from build123d import *

# Parameters (mm, degrees)
SKETCH_R        = 25
PAD_DEPTH       = 25
PAD_TAPER       = 15
SKETCH001_R     = 22.984215
POCKET_DEPTH    = 17
POCKET_TAPER    = 15
SKETCH002_R     = 16.714516
PAD001_DEPTH    = 30
PAD001_TAPER    = 20
SKETCH003_R     = 4.228339
POCKET001_DEPTH = 20


with BuildPart() as part:
    # Sketch → Pad (new body)
    with BuildSketch(Plane.XY):
        Circle(SKETCH_R)
    extrude(amount=PAD_DEPTH, taper=PAD_TAPER)

    # Sketch001 (on Face2 of Pad) → Pocket (cut)
    with BuildSketch(Plane(origin=(0, 0, 0), x_dir=(1, 0, 0), z_dir=(0, 0, -1))):
        Circle(SKETCH001_R)
    extrude(amount=-POCKET_DEPTH, taper=POCKET_TAPER, mode=Mode.SUBTRACT)

    # Sketch002 (on Face5 of Pocket) → Pad001 (join)
    with BuildSketch(Plane(origin=(0, 0, 17), x_dir=(1, 0, 0), z_dir=(0, 0, -1))):
        Circle(SKETCH002_R)
    extrude(amount=PAD001_DEPTH, taper=PAD001_TAPER)

    # Sketch003 (on Face7 of Pad001) → Pocket001 (cut)
    with BuildSketch(Plane(origin=(0, 0, -13), x_dir=(1, 0, 0), z_dir=(0, 0, -1))):
        Circle(SKETCH003_R)
    extrude(amount=-POCKET001_DEPTH, mode=Mode.SUBTRACT)


solid = part.part
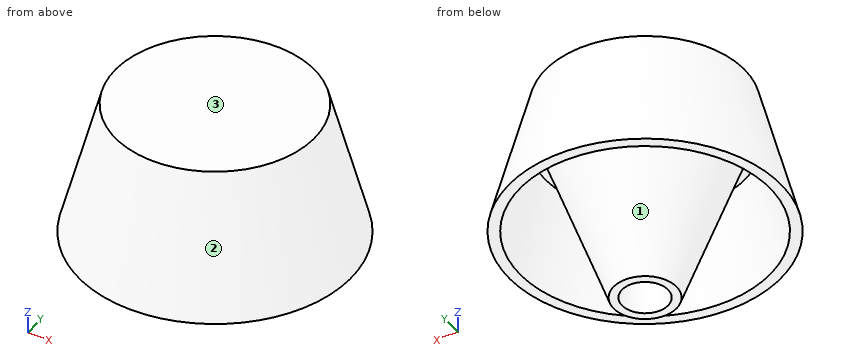
Could you check a few things on this model? Use its own coordinates, in mm. Face numbers are marked on the shaded views. Give positions to 0.01 mm unless a question says otherwise; leave off trailing zeros. Order: outer loops, then holes, each group sorted by start corner. A loop starts at its lowest first (then second) coordinate and runs counter-clockwise, first axis right, second up. Notation, with made-up numbers: (36, 82.25) - (77, 82.25) arc R23 ccw to (77, 94.25) - close; hole circle Ø11 at (68.5, -16.5). An arc over 180 degrees is marked (long way). One line per question, with ' | ' between items. Start each with the question number.
Item 1: Thinking about a two-plate mould opening in X: for the marked faces 1, 2 and 3, which applies, pulls with the +X half, pulls with the -X half, needs draft (parallel to the pull), parting line crosses it, or undercut?
Item 2: I want a section at C-C on z = -1.5. Write out the boundary of the cut face in (x, y).
Item 3: I want a section at A-A on x = 0. Write out the boundary of the cut face in (y, z).
Item 4: I'm going to push flat-ended pins straight in: pin 1 Ø6 at (y, z) = (3, 18) entering from -X; pin 2 Ø8 at (x, z) = (9.5, 0.5) entering from +Y; pin 3 Ø5 at (x, z) = (-7.5, -5.5) entering from +Y. Where does each tip first touch, or does it pass through?
Item 5: I want a section at B-B on z = 4. Write out the boundary of the cut face in (x, y).
Item 6: I need wall thicknesses on probe 1 along Y at (x, z) = (-8, 16); probe 2 along X at (y, z) = (9.5, 8); probe 3 along Y at (x, z) = (8, 13.5). Which ranges of each line are inside material? Lowest first, please. Write a range as [from, to].
Item 7: I want a section at D-D on z = 19. Write out the boundary of the cut face in (x, y), then the cut area to 3 significant figures.
Verdict:
1) face 1: undercut | face 2: parting line crosses it | face 3: needs draft
2) outline: circle Ø19.96 at (0, 0); hole circle Ø8.46 at (0, 0)
3) outline: (-25, 0) - (-22.98, 0) - (-18.43, 17) - (-16.71, 17) - (-5.8, -13) - (-4.23, -13) - (-4.23, 7) - (4.23, 7) - (4.23, -13) - (5.8, -13) - (16.71, 17) - (18.43, 17) - (22.98, 0) - (25, 0) - (18.3, 25) - (-18.3, 25) - close
4) pin 1: x = -20.84 | pin 2: y = 24.38 | pin 3: y = 7.22
5) outline: circle Ø47.86 at (0, 0); circle Ø23.97 at (0, 0); hole circle Ø43.82 at (0, 0); hole circle Ø8.46 at (0, 0)
6) probe 1: [-19.11, -16.9], [-14.26, 14.26], [16.9, 19.11] | probe 2: [-20.79, -18.55], [-9.51, 9.51], [18.55, 20.79] | probe 3: [-19.83, -17.64], [-13.21, 13.21], [17.64, 19.83]
7) outline: circle Ø39.82 at (0, 0) | area: 1,250 mm^2
